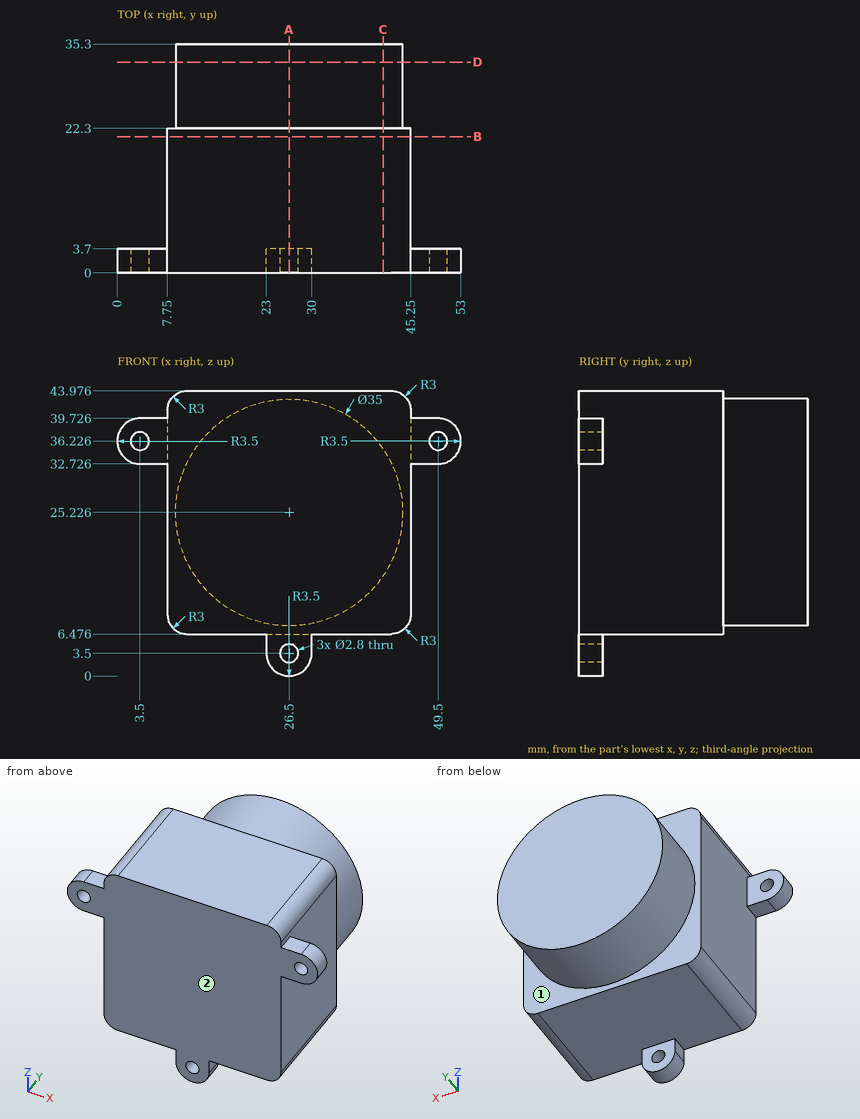
Design review of the part shown in the three views and the two pictorial views. Dimensions are in mm from the part's minimum x, y and z. A direction names the side the tool comes from. Round coordinates to 2 decimals unless told otherwise and drop trailing zeros. Order: outer loops, then holes, each group sorted by start corner. A loop starts at its lowest first (then second) coordinate and runs counter-clockwise, first axis right, second up.
Q1. Wall thickness on line 1 (Z direction, x = 3.5, y = 2.4); line 2 (Z direction, x = 26.5, y = 2.8); line 3 (Z direction, x = 33, y = 2.5): over which ranges is each line inside the solid? List them lowest first.
Findings below:
line 1: z = 32.73 to 34.83, 37.63 to 39.73
line 2: z = 0 to 2.1, 4.9 to 43.98
line 3: z = 6.48 to 43.98
Q2. Machinability: for the marked faces 1 and 2, which of the approach directions +Z, -Z, +X, -X, +Y, -Y give a long, thin tool a straight path to every point of the face, cutting with its end or side? Answer none if there is none.
Findings below:
face 1: +Y
face 2: +Z, -Z, +X, -X, -Y
Q3. We need section B-B, the plane y = 21. Give the boundary of the cut face in (x, z), plus the area to 3 significant figures.
Findings below:
outline: (7.75, 9.48) arc R3 ccw to (10.75, 6.48) - (42.25, 6.48) arc R3 ccw to (45.25, 9.48) - (45.25, 40.98) arc R3 ccw to (42.25, 43.98) - (10.75, 43.98) arc R3 ccw to (7.75, 40.98) - close
area: 1,400 mm2
Q4. Insertion check: P1, Ø18, axis at y = 10, z = 23, coming from the -X side; P2, Ø2, axis at x = 26.5, z = 3.5, coming from the -Y side; P3, Ø2.5, axis at y = 2, z = 4.5, coming from the +X side; P4, Ø6.5, axis at y = 11.5, z = 27, coming from the +X side. Each pin has a flat end and moves straight along its axis. Give the tip position at first contact, or say it passes through.
Findings below:
P1: stops at x = 7.75
P2: passes through
P3: stops at x = 30
P4: stops at x = 45.25
Q5. We need section C-C, the plane x = 41. Give the boundary of the cut face in (y, z), plus the area to 3 significant figures.
Findings below:
outline: (0, 6.48) - (22.3, 6.48) - (22.3, 15.43) - (35.3, 15.43) - (35.3, 35.02) - (22.3, 35.02) - (22.3, 43.98) - (0, 43.98) - close
area: 1,090 mm2
Q6. We need section D-D, the plane y = 32.5. Give the boundary of the cut face in (x, z).
Findings below:
outline: circle Ø35 at (26.5, 25.23)
Q7. We need section A-A, the plane x = 26.5. Give the boundary of the cut face in (y, z).
Findings below:
outline: (0, 0) - (3.7, 0) - (3.7, 2.1) - (0, 2.1) - close; (0, 4.9) - (3.7, 4.9) - (3.7, 6.48) - (22.3, 6.48) - (22.3, 7.73) - (35.3, 7.73) - (35.3, 42.73) - (22.3, 42.73) - (22.3, 43.98) - (0, 43.98) - close
